from build123d import *

# Parameters (mm, degrees)
F1_DEPTH = 12
F2_R     = 5
F3_R     = 2.2
F4_DEPTH = 40.001
F6_START = -5
F6_DEPTH = 35.0010001


with BuildPart() as f1:
    # F0 (on Right) → F1 (new body)
    with BuildSketch(Plane.YZ):
        with BuildLine():
            Line((0, -40), (0, 0))
            Line((0, 0), (-120, 0))
            Line((-120, 0), (-120, -5.6517750396))
            ThreePointArc((-120, -5.6517750396), (-118.2666855434, -10.6245662378), (-113.8178369249, -13.4425047175))
            Line((-113.8178369249, -13.4425047175), (0, -40))
        make_face()
    extrude(amount=F1_DEPTH)

    # F2
    f2_edges = [f1.edges().sort_by_distance(p)[0] for p in [
        (0, -56.908918, -26.721252),
        (12, -56.908918, -26.721252),
    ]]
    fillet(f2_edges, radius=F2_R)

    # F3 (on face) → F4 (cut, through all)
    with BuildSketch(Plane.XY):
        with Locations((6, -30)):
            Circle(F3_R)
        with Locations((6, -90)):
            Circle(F3_R)
    extrude(amount=-F4_DEPTH, mode=Mode.SUBTRACT)

    # F5 (on face) → F6 (cut)
    with BuildSketch(Plane.XY.offset(F6_START)):
        Polygon((2.45, -32.0495934556), (6, -34.0991869112), (9.55, -32.0495934556), (9.55, -27.9504065444), (6, -25.9008130888), (2.45, -27.9504065444), align=None)
        Polygon((2.45, -92.0495934556), (6, -94.0991869112), (9.55, -92.0495934556), (9.55, -87.9504065444), (6, -85.9008130888), (2.45, -87.9504065444), align=None)
    extrude(amount=-F6_DEPTH, mode=Mode.SUBTRACT)


solid = f1.part
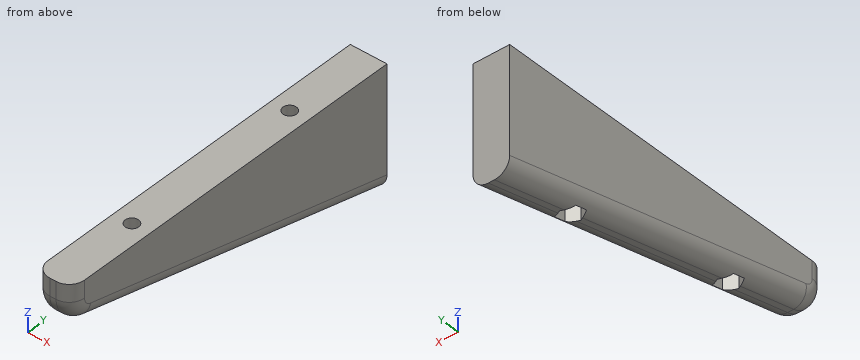
Can you work these out from the model? Positions are in its coordinate system, mm. Give positions to 0.01 mm unless a question says otherwise; leave off trailing zeros. Loops run counter-clockwise (first coordinate to the right, second up) from the corner with the lowest first, then second, coordinate; pieces in that order, holes last. Notation, with made-up numbers: M 30.5,50 L 69.5,50 A30 ccw 69.5,87 Z; hole C 72,48.5 d5. An arc over 180 degrees is marked long. One line per item, written item: value.
1) Imagine slicing it at A-A on z = -2. Write out the boundary of the cut face in (x, y).
Geometry check:
outline: M 0,-115 A5 ccw 5,-120 L 7,-120 A5 ccw 12,-115 L 12,0 L 0,0 Z; hole C 6,-90 d4.4; hole C 6,-30 d4.4
2) Imagine slicing it at B-B on z = -15.5. Count the separate pieces of the cut face and the enclosed holes in it, and give its area (3 significant figures).
Geometry check:
separate pieces: 1
enclosed holes: 2
area: 1,130 mm²
3) I'm going to push flat-ended pins straight in: pin 1 (1 mm diameter, centred on x = 6, y = -92, fed in from -Z); pin 2 (1.5 mm diameter, centred on x = 8.5, z = -13, fed in from -Y); pin 3 (5.5 mm diameter, centred on x = 7.5, y = -88.5, fed in from -Z). Where does each tip first touch, or does it pass through?
Geometry check:
pin 1: stops at z = -5
pin 2: stops at y = -116.17
pin 3: stops at z = -19.98
4) Please list where these lines run through material, in increasing order: line 1 (Y direction, x = 6, z = -2.7); line 2 (X direction, y = -29.5, z = -24); line 3 (X direction, y = -94, z = -12).
Geometry check:
line 1: y = -120 to -92.2, -87.8 to -32.2, -27.8 to 0
line 2: x = 0 to 2.45, 9.55 to 12
line 3: x = 0 to 5.83, 6.17 to 12
